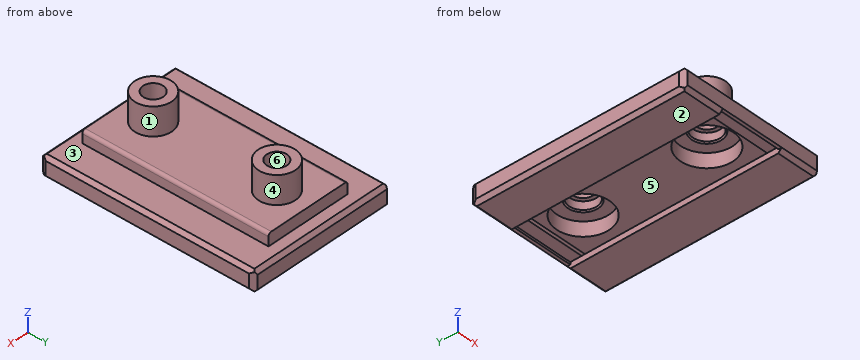
from build123d import *
from OCP.BRepFilletAPI import BRepFilletAPI_MakeChamfer

# Parameters (mm, degrees)
SKETCH1_W           = 23.9
SKETCH1_H           = 34.7
BOSS_EXTRUDE1_DEPTH = 3.4
SKETCH2_W           = 14
SKETCH2_H           = 30.1
BOSS_EXTRUDE2_DEPTH = 1.95
SKETCH3_R           = 3
BOSS_EXTRUDE3_DEPTH = 4.5
CHAMFER1_SIZE       = 0.577
CUT_EXTRUDE1_DEPTH  = 5.2
SKETCH6_W           = 14
SKETCH6_H           = 30
CUT_EXTRUDE2_DEPTH  = 0.6
SKETCH7_R           = 4.25
CUT_EXTRUDE3_DEPTH  = 2.3
SKETCH8_R           = 2.25
CUT_EXTRUDE4_DEPTH  = 1.5
FILLET1_R           = 0.5
CHAMFER2_SIZE       = 0.577
CHAMFER3_SIZE       = 0.527
CHAMFER3_SIZE2      = 0.913344887
CHAMFER4_SIZE       = 0.913344887
CHAMFER4_SIZE2      = 0.527
CUT_EXTRUDE5_REACH  = 25.256
SKETCH9_R           = 1.621
CHAMFER5_SIZE       = 0.2


with BuildPart() as part:
    # Sketch1 → Boss-Extrude1 (new body)
    with BuildSketch(Plane.XY):
        Rectangle(SKETCH1_W, SKETCH1_H)
    extrude(amount=-BOSS_EXTRUDE1_DEPTH)

    # Sketch2 → Boss-Extrude2 (add)
    with BuildSketch(Plane.XY):
        Rectangle(SKETCH2_W, SKETCH2_H)
    extrude(amount=BOSS_EXTRUDE2_DEPTH)

    # Sketch3 → Boss-Extrude3 (add)
    with BuildSketch(Plane.XY.offset(1.95)):
        with Locations(Location((0, 10, 0), (0, 0, 180))):
            Circle(SKETCH3_R)
        with Locations(Location((0, -10, 0), (0, 0, 180))):
            Circle(SKETCH3_R)
    extrude(amount=BOSS_EXTRUDE3_DEPTH)

    # Chamfer1
    chamfer1_edges = [part.edges().sort_by_distance(p)[0] for p in [
        (11.95, 0, -3.4),
        (0, 17.35, -3.4),
        (-11.95, 0, -3.4),
        (0, -17.35, -3.4),
    ]]
    chamfer(chamfer1_edges, length=CHAMFER1_SIZE)

    # Sketch5 → Cut-Extrude1 (cut, symmetric)
    with BuildSketch(Plane(origin=(0, 0, 0), x_dir=(0, 0, -1), z_dir=(1, 0, 0))):
        Polygon((3.4, 16.773), (2.823, 17.35), (2.823, 16.826999997), (2.449999998, 16.826999997), (2.449999998, -16.826999997), (2.823, -16.826999997), (2.823, -17.35), (3.4, -16.773), align=None)
    extrude(amount=CUT_EXTRUDE1_DEPTH, both=True, mode=Mode.SUBTRACT)

    # Sketch6 → Cut-Extrude2 (cut)
    with BuildSketch(Plane(origin=(0, 0, -2.449999998), x_dir=(-1, 0, 0), z_dir=(0, 0, -1))):
        Rectangle(SKETCH6_W, SKETCH6_H)
    extrude(amount=-CUT_EXTRUDE2_DEPTH, mode=Mode.SUBTRACT)

    # Sketch7 → Cut-Extrude3 (cut)
    with BuildSketch(Plane.XY.offset(-1.849999998)):
        with Locations(Location((0, 10, 0), (0, 0, 180))):
            Circle(SKETCH7_R)
        with Locations(Location((0, -10, 0), (0, 0, 180))):
            Circle(SKETCH7_R)
    extrude(amount=CUT_EXTRUDE3_DEPTH, mode=Mode.SUBTRACT)

    # Sketch8 → Cut-Extrude4 (cut)
    with BuildSketch(Plane.XY.offset(0.450000002)):
        with Locations(Location((0, 10, 0), (0, 0, 180))):
            Circle(SKETCH8_R)
        with Locations(Location((0, -10, 0), (0, 0, 180))):
            Circle(SKETCH8_R)
    extrude(amount=CUT_EXTRUDE4_DEPTH, mode=Mode.SUBTRACT)

    # Fillet1
    fillet1_edges = [part.edges().sort_by_distance(p)[0] for p in [
        (-7, 0, 1.95),
        (7, 0, 1.95),
    ]]
    fillet(fillet1_edges, radius=FILLET1_R)

    # Chamfer2
    chamfer2_edges = [part.edges().sort_by_distance(p)[0] for p in [
        (0, 17.35, 0),
        (11.95, 0, 0),
        (0, -17.35, 0),
        (-11.95, 0, 0),
    ]]
    chamfer(chamfer2_edges, length=CHAMFER2_SIZE)

    # Chamfer3: one chamfer whose edges measure the first distance from different faces: ONE call of the kernel's chamfer builder (chamfer() names one face for all edges)
    chamfer3_edges_1 = [part.edges().sort_by_distance(p)[0] for p in [
        (11.95, 17.35, -1.7),
    ]]
    chamfer3_side_1 = [part.faces().sort_by_distance(p)[0] for p in [
        (0, 17.35, -1.7),
    ]]
    chamfer3_edges_2 = [part.edges().sort_by_distance(p)[0] for p in [
        (-11.95, -17.35, -1.7),
    ]]
    chamfer3_side_2 = [part.faces().sort_by_distance(p)[0] for p in [
        (0, -17.35, -1.7),
    ]]
    chamfer3 = BRepFilletAPI_MakeChamfer(part.part.solid().wrapped)
    for e in chamfer3_edges_1:
        chamfer3.Add(CHAMFER3_SIZE, CHAMFER3_SIZE2, e.wrapped, chamfer3_side_1[0].wrapped)  # the first distance lies on this face
    for e in chamfer3_edges_2:
        chamfer3.Add(CHAMFER3_SIZE, CHAMFER3_SIZE2, e.wrapped, chamfer3_side_2[0].wrapped)  # the first distance lies on this face
    add(Compound.cast(chamfer3.Shape()), mode=Mode.REPLACE)

    # Chamfer4: one chamfer whose edges measure the first distance from different faces: ONE call of the kernel's chamfer builder (chamfer() names one face for all edges)
    chamfer4_edges_1 = [part.edges().sort_by_distance(p)[0] for p in [
        (-11.95, 17.35, -1.7),
    ]]
    chamfer4_side_1 = [part.faces().sort_by_distance(p)[0] for p in [
        (-11.95, 0.456672443, -1.7),
    ]]
    chamfer4_edges_2 = [part.edges().sort_by_distance(p)[0] for p in [
        (11.95, -17.35, -1.7),
    ]]
    chamfer4_side_2 = [part.faces().sort_by_distance(p)[0] for p in [
        (11.95, -0.456672443, -1.7),
    ]]
    chamfer4 = BRepFilletAPI_MakeChamfer(part.part.solid().wrapped)
    for e in chamfer4_edges_1:
        chamfer4.Add(CHAMFER4_SIZE, CHAMFER4_SIZE2, e.wrapped, chamfer4_side_1[0].wrapped)  # the first distance lies on this face
    for e in chamfer4_edges_2:
        chamfer4.Add(CHAMFER4_SIZE, CHAMFER4_SIZE2, e.wrapped, chamfer4_side_2[0].wrapped)  # the first distance lies on this face
    add(Compound.cast(chamfer4.Shape()), mode=Mode.REPLACE)

    # Sketch9 → Cut-Extrude5 (cut, up to next)
    with BuildSketch(Plane.XY.offset(6.45), mode=Mode.PRIVATE) as cut_extrude5_sk1:
        with Locations((0, 10)):
            Circle(SKETCH9_R)
    cut_extrude5_tool1 = extrude(cut_extrude5_sk1.sketch, amount=-CUT_EXTRUDE5_REACH, mode=Mode.PRIVATE) & part.part
    # Sketch9 → Cut-Extrude5 (cut, up to next)
    with BuildSketch(Plane.XY.offset(6.45), mode=Mode.PRIVATE) as cut_extrude5_sk2:
        with Locations((0, -10)):
            Circle(SKETCH9_R)
    cut_extrude5_tool2 = extrude(cut_extrude5_sk2.sketch, amount=-CUT_EXTRUDE5_REACH, mode=Mode.PRIVATE) & part.part
    add(cut_extrude5_tool1.solids().sort_by_distance((0, 10, 6.45))[0], mode=Mode.SUBTRACT)
    add(cut_extrude5_tool2.solids().sort_by_distance((0, -10, 6.45))[0], mode=Mode.SUBTRACT)

    # Chamfer5
    chamfer5_edges = [part.edges().sort_by_distance(p)[0] for p in [
        (2.25, -10, 0.450000002),
        (2.25, 10, 0.450000002),
    ]]
    chamfer(chamfer5_edges, length=CHAMFER5_SIZE)


solid = part.part
Geometry: final body of the model. Coordinates: model frame, mm. Face numbers are marked on the shaded views. A direction names the side the tool comes from. Give positions to 0.01 mm unless a question says otherwise; leave off trailing zeros. Loops run counter-clockwise (first coordinate to the right, second up) from the corner with the lowest first, then second, coordinate; pieces in that order, holes last. Notation, with made-up numbers: M 74,20 L 109,20 A26 ccw 109,52 Z; hole C -26,28 d9. An arc over 180 degrees is marked long. Put each result on its own line as item: value. Start each with the question number.
1) Cut plane A-A (x = -5.75). Output: boundary loops of the cut face in (y, z), then the cut area to 3 significant figures.
2) Contact query for flat-ended pins moving along their axis: pin 1 (1 mm diameter, centred on x = -3.5, y = -13.5, fed in from -Z); pin 2 (1.2 mm diameter, centred on y = 4.5, z = 0.5, fed in from +X); pin 3 (2.5 mm diameter, centred on x = 0, y = -10, fed in from +Z); pin 4 (1.3 mm diameter, centred on x = -1, y = -10.5, fed in from -Z). Output: stop coordinate, or through.
3) Cut plane C-C (z = -1). Output: boundary loops of the cut face in (x, y), then the cut area to 3 significant figures.
4) Cut plane B-B (y = 4.5). Output: boundary loops of the cut face in (x, z).
5) Pull-direction query (X, two-part tool) for the marked faces 3, 4, 5 and 6; classes: pulls with the +X half, pulls with the -X half, needs draft (parallel to the pull), parting line crosses it, or undercut.
6) Cut plane D-D (x = 0). Give the number of separate pieces and of enclosed holes in the cut face, then the cut area to 3 significant figures.
7) Access query for the marked faces 1 and 2. Directions: +Z, -Z, +X, -X, +Y, -Y. A direction counts if a zero-diameter tool reaches every point of the face in a straight line with its end or side. Return the directions, or none.
8) Ray query, line 1 along Y through (x, z) = (0, 1.15); line 2 along Y through (x, z) = (0, 3.55); line 3 along Z through (x, y) = (-5.25, 8). Return the intervals inside material, ascending.
Verdict:
1. outline: M -17.35,-2.82 L -16.77,-3.4 L 16.77,-3.4 L 17.35,-2.82 L 17.35,-0.58 L 16.77,0 L 15.05,0 L 15.05,1.95 L -15.05,1.95 L -15.05,0 L -16.77,0 L -17.35,-0.58 Z; hole M -15,-2.45 L 15,-2.45 L 15,-1.85 L -15,-1.85 Z
1. area: 158 mm2
2. pin 1: z = -1.85
2. pin 2: x = 11.47
2. pin 3: through
2. pin 4: z = 1.95
3. outline: M -11.95,-16.44 L -11.42,-17.35 L 11.42,-17.35 L 11.95,-16.44 L 11.95,16.44 L 11.42,17.35 L -11.42,17.35 L -11.95,16.44 Z; hole C 0,-10 d8.5; hole C 0,10 d8.5
3. area: 715 mm2
4. outline: M -11.95,-2.82 L -11.37,-3.4 L -5.2,-3.4 L -5.2,-2.45 L -7,-2.45 L -7,-1.85 L 7,-1.85 L 7,-2.45 L 5.2,-2.45 L 5.2,-3.4 L 11.37,-3.4 L 11.95,-2.82 L 11.95,-0.58 L 11.37,0 L 7,0 L 7,1.45 A0.5 ccw 6.5,1.95 L -6.5,1.95 A0.5 ccw -7,1.45 L -7,0 L -11.37,0 L -11.95,-0.58 Z
5. face 3: needs draft
5. face 4: parting line crosses it
5. face 5: undercut
5. face 6: undercut
6. separate pieces: 3
6. enclosed holes: 0
6. area: 97.9 mm2
7. face 1: +Z
7. face 2: -Z, +X, -X, +Y, -Y
8. line 1: -15.05 to -12.25, -7.75 to 7.75, 12.25 to 15.05
8. line 2: -13 to -11.62, -8.38 to -7, 7 to 8.38, 11.62 to 13
8. line 3: -3.4 to -2.45, -1.85 to 1.95
